Input: dimensioned drawing with shaded views. Units: mm. Origin: part minimum x, y, z. Give positions to 0.01 mm unless a question says otherwise; leave off trailing zeros. Loops run counter-clockwise (first coordinate to the right, second up) from the corner with the lowest first, then second, coordinate; pieces in that order, holes last. Notation, with made-up numbers: (53, 88.5) -> (93, 88.5) arc R22 cw to (93, 115.5) -> close; hole circle Ø9 at (-31.5, 58.25). An arc over 180 degrees is marked (long way). Answer in a Markdown table with one row per item. Add a question column.
1) Section query A-A (z = 54.5). Return the cut outline in (x, y), plus the area to 3 significant figures.
2) Section query B-B (x = 30). Return the cut outline in (y, z), plus the area to 3 significant figures.
3) Line query: line 1 (Z direction, x = 23.5, y = 1.7); line 2 (X direction, y = 2.9, z = 17); line 3 (Z direction, x = 26.5, y = 3.45) (1 decimal). Output: solid intervals per line, ascending. Write a range as from..to.
4) First-contact query: P1, Ø2.5, axis at y = 3, z = 100.5, coming from the -X side; P2, Ø3.5, axis at x = 35.08, z = 64.66, coming from the -Y side; P3, Ø2.5, axis at y = 3.5, z = 99, coming from the +X side; P4, Ø1.5, axis at x = 29.5, y = 1.5, coming from the -Z side. Flat tips, straight axial feed; report the tip coordinate or a pass-through.
5) Section query D-D (x = 46.5). Return the cut outline in (y, z) (3 decimals), plus the area to 3 significant figures.
6) Section query C-C (y = 4.15). Return the cut outline in (x, z) (3 decimals), plus the area to 3 significant figures.
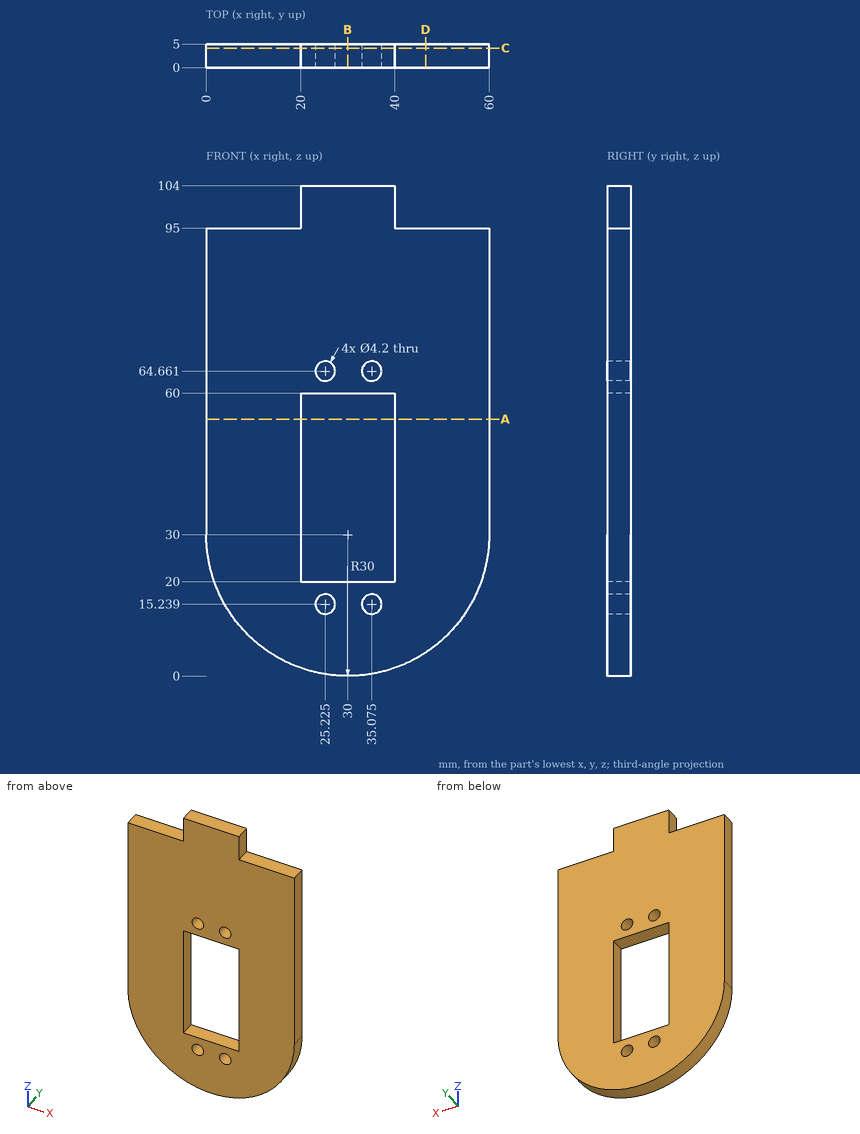
Evaluation:
| question | item | result |
|---|---|---|
| 1 | outline | (0, 0) -> (20, 0) -> (20, 5) -> (0, 5) -> close; (40, 0) -> (60, 0) -> (60, 5) -> (40, 5) -> close |
| 1 | area | 200 mm² |
| 2 | outline | (0, 0) -> (5, 0) -> (5, 20) -> (0, 20) -> close; (0, 60) -> (5, 60) -> (5, 104) -> (0, 104) -> close |
| 2 | area | 320 mm² |
| 3 | line 1 | 0.71..14.04, 16.44..20, 60..63.46, 65.86..104 |
| 3 | line 2 | 2.96..24.08, 26.37..33.93, 36.22..57.04 |
| 3 | line 3 | 0.2..13.6, 16.9..20, 60..63, 66.3..104 |
| 4 | P1 | x = 20 |
| 4 | P2 | through |
| 4 | P3 | x = 40 |
| 4 | P4 | z = 0 |
| 5 | outline | (0, 4.945) -> (5, 4.945) -> (5, 95) -> (0, 95) -> close |
| 5 | area | 450 mm² |
| 6 | outline | (0, 30) arc R30 ccw to (60, 30) -> (60, 95) -> (40, 95) -> (40, 104) -> (20, 104) -> (20, 95) -> (0, 95) -> close; hole (20, 20) -> (40, 20) -> (40, 60) -> (20, 60) -> close; hole circle Ø4.2 at (25.225, 15.239); hole circle Ø4.2 at (25.225, 64.661); hole circle Ø4.2 at (35.075, 15.239); hole circle Ø4.2 at (35.075, 64.661) |
| 6 | area | 4,640 mm² |
